Input: part model. Units: mm. Frame: model coordinates. Coordinates: 2 decimals unless noted, no trailing zeros. Order: outer loops, then holes, each group sorted by start corner. A loop starts at its lowest first (then second) coordinate and runs counter-clockwise, first axis right, second up. Notation, with made-up numbers: (72, 43) -> (100, 43) arc R17 ccw to (100, 69) -> close; hole circle Ø3 at (55.5, 85). An arc over 180 degrees is marked (long way). Use one line per item in the form item = value. Start each with the question number.
1) Pin query (flat end, axial travel): pin 1 (5.5 mm diameter, centred on x = 328.79, y = -30.47, fed in from -Z); pin 2 (3 mm diameter, centred on x = -278, z = 3, fed in from +Y). Return the tip coordinate at first contact, or that it passes through.
2) Section query C-C on z = 5. Count the separate pieces of the cut face and the enclosed holes in it, then the cut area to 3 significant figures.
3) Ray query, line 1 along Y through (x, z) = (-6.5, 1.5); line 2 along Y through (x, z) = (171.5, 5); line 3 along Y through (x, z) = (-8, 5). Return the intervals inside material, ascending.
4) Section query D-D on y = 265.5. Output: boundary loops of the cut face in (x, z).
5) Section query A-A on y = 0. Output: boundary loops of the cut face in (x, z), then the cut area to 3 significant figures.
6) Section query B-B on x = -96.5. Output: boundary loops of the cut face in (y, z).
7) Draft query along X for faces 1 (the flat face through (-242, 84, 6.35)), 2 (the cylindrical face through (339.18, -106.81, 3.13)), 3 (the cylindrical face through (-55.06, 247.96, 3.13)). Return one class per face: pulls with the +X half, pulls with the -X half, needs draft (parallel to the pull), parting line crosses it, or undercut.
Autodesk Inventor part; units mm, degrees
ref_plane "YZ Plane" through (0, 0, 0) normal (1, 0, 0) x (0, 1, 0)
ref_plane "XZ Plane" through (0, 0, 0) normal (0, 1, 0) x (-1, 0, 0)
ref_plane "XY Plane" through (0, 0, 0) normal (0, 0, 1) x (1, 0, 0)
sketch "Sketch1" plane through (0, 0, 0) normal (0, 0, 1) x (1, 0, 0)
  circle A0 centre (0, 0) radius 355.6
  circle A1 centre (0, 0) radius 254
  circle A2 centre (0, -330.2) radius 3.175
  circle A3 centre (119.282, -307.9023) radius 3.175
  circle A4 centre (222.4543, -244.0207) radius 3.175
  circle A5 centre (295.5829, -147.1828) radius 3.175
  circle A6 centre (328.7914, -30.467) radius 3.175
  circle A7 centre (317.5948, 90.3635) radius 3.175
  circle A8 centre (263.5053, 198.99) radius 3.175
  circle A9 centre (173.8279, 280.7417) radius 3.175
  circle A10 centre (60.6741, 324.5777) radius 3.175
  circle A11 centre (-60.6741, 324.5777) radius 3.175
  circle A12 centre (-173.8279, 280.7417) radius 3.175
  circle A13 centre (-263.5053, 198.99) radius 3.175
  circle A14 centre (-317.5948, 90.3635) radius 3.175
  circle A15 centre (-328.7914, -30.467) radius 3.175
  circle A16 centre (-295.5829, -147.1828) radius 3.175
  circle A17 centre (-222.4543, -244.0207) radius 3.175
  circle A18 centre (-119.282, -307.9023) radius 3.175
  dimension "d0" = 711.2
  dimension "d1" = 508
  dimension "d3" = 6.35
  dimension "d6" = 360
extrude "Extrusion1" add sketch "Sketch1" along normal blind 6.35
properties part number "back layer of front"
Answers below:
q1.pin_1 = through
q1.pin_2 = 223.6
q2.separate_pieces = 1
q2.enclosed_holes = 18
q2.area = 194,000 mm^2
q3.line_1 = -355.54 to -253.92, 253.92 to 355.54
q3.line_2 = -311.51 to -187.36, 187.36 to 278.58, 282.9 to 311.51
q3.line_3 = -355.51 to -253.87, 253.87 to 355.51
q4.outline = (-236.56, 0) -> (236.56, 0) -> (236.56, 6.35) -> (-236.56, 6.35) -> close
q5.outline = (-355.6, 0) -> (-254, 0) -> (-254, 6.35) -> (-355.6, 6.35) -> close; (254, 0) -> (355.6, 0) -> (355.6, 6.35) -> (254, 6.35) -> close
q5.area = 1,290 mm^2
q6.outline = (-342.26, 0) -> (-234.95, 0) -> (-234.95, 6.35) -> (-342.26, 6.35) -> close; (234.95, 0) -> (342.26, 0) -> (342.26, 6.35) -> (234.95, 6.35) -> close
q7.face_1 = needs draft
q7.face_2 = parting line crosses it
q7.face_3 = undercut
